from build123d import *

# Parameters (mm, degrees)
ESQUISSE1_R             = 24
BOSS_EXTRU_1_DEPTH      = 14
BOSS_EXTRU_2_DEPTH      = 8
ESQUISSE3_R             = 1.75
ENL_V_MAT_EXTRU_1_DEPTH = 8
BOSS_EXTRU_3_DEPTH      = 40
ESQUISSE5_R             = 17
BOSS_EXTRU_4_DEPTH      = 28
ESQUISSE6_R             = 13
ENL_V_MAT_EXTRU_2_DEPTH = 4
CHANFREIN1_SIZE         = 1


with BuildPart() as part:
    # Esquisse1 → Boss.-Extru.1 (new body)
    with BuildSketch(Plane(origin=(0, 0, 0), x_dir=(0, 0, -1), z_dir=(1, 0, 0))):
        Circle(ESQUISSE1_R)
    extrude(amount=BOSS_EXTRU_1_DEPTH)

    # Esquisse2 → Boss.-Extru.2 (add)
    with BuildSketch(Plane(origin=(14, 0, 0), x_dir=(0, 0, -1), z_dir=(1, 0, 0))):
        with BuildLine():
            Line((-32, -24), (32, -24))
            ThreePointArc((32, -24), (36.242640687, -22.242640687), (38, -18))
            Line((38, -18), (38, 18))
            ThreePointArc((38, 18), (36.242640687, 22.242640687), (32, 24))
            Line((32, 24), (-32, 24))
            ThreePointArc((-32, 24), (-36.242640687, 22.242640687), (-38, 18))
            Line((-38, 18), (-38, -18))
            ThreePointArc((-38, -18), (-36.242640687, -22.242640687), (-32, -24))
        make_face()
    extrude(amount=BOSS_EXTRU_2_DEPTH)

    # Esquisse3 → Enlèv. mat.-Extru.1 (cut)
    with BuildSketch(Plane(origin=(22, 0, 0), x_dir=(0, 0, -1), z_dir=(1, 0, 0))):
        with Locations((31, 17)):
            Circle(ESQUISSE3_R)
        with Locations((-31, 17)):
            Circle(ESQUISSE3_R)
        with Locations((-31, -17)):
            Circle(ESQUISSE3_R)
        with Locations((31, -17)):
            Circle(ESQUISSE3_R)
    extrude(amount=-ENL_V_MAT_EXTRU_1_DEPTH, mode=Mode.SUBTRACT)

    # Esquisse4 → Boss.-Extru.3 (add)
    with BuildSketch(Plane(origin=(22, 0, 0), x_dir=(0, 0, -1), z_dir=(1, 0, 0))):
        with BuildLine():
            Line((-22, -20), (22, -20))
            ThreePointArc((22, -20), (25.535533906, -18.535533906), (27, -15))
            Line((27, -15), (27, 15))
            ThreePointArc((27, 15), (25.535533906, 18.535533906), (22, 20))
            Line((22, 20), (-22, 20))
            ThreePointArc((-22, 20), (-25.535533906, 18.535533906), (-27, 15))
            Line((-27, 15), (-27, -15))
            ThreePointArc((-27, -15), (-25.535533906, -18.535533906), (-22, -20))
        make_face()
    extrude(amount=BOSS_EXTRU_3_DEPTH)

    # Esquisse5 → Boss.-Extru.4 (add)
    with BuildSketch(Plane(origin=(62, 0, 0), x_dir=(0, 0, -1), z_dir=(1, 0, 0))):
        Circle(ESQUISSE5_R)
    extrude(amount=BOSS_EXTRU_4_DEPTH)

    # Esquisse6 → Enlèv. mat.-Extru.2 (cut)
    with BuildSketch(Plane(origin=(90, 0, 0), x_dir=(0, 0, -1), z_dir=(1, 0, 0))):
        Circle(ESQUISSE6_R)
    extrude(amount=-ENL_V_MAT_EXTRU_2_DEPTH, mode=Mode.SUBTRACT)

    # Chanfrein1
    chanfrein1_edges = [part.edges().sort_by_distance(p)[0] for p in [
        (90, 0, 17),
    ]]
    chamfer(chanfrein1_edges, length=CHANFREIN1_SIZE)


solid = part.part
Could you check a few things on this model? Use its own coordinates, in mm. A direction names the side the tool comes from. Give positions to 0.01 mm unless a question says otherwise; leave off trailing zeros. Write each loop counter-clockwise with the first axis right and the second up, starting at its lowest first coordinate (ties: lowest second). Pieces come first, ordered by that corner, then holes. Notation, with made-up numbers: (-8, 77.25) - (19, 77.25) arc R19 cw to (19, 84.25) - close; hole circle Ø9 at (42, 89). An arc over 180 degrees is marked (long way). Use CSV: the item, a comma, the result in double quotes. Start each with the question number.
Item 1: For faces 1 (the face through (86, 0, 0)), 2 (the face through (42, 0, -27)), 3 (the face through (14, 0, 28)), which set-ups out of +Z, -Z, +X, -X, +Y, -Y let a thin tool reach every point of the face, with its end or its side?
Item 2: If I drill on line 1 along Y through (x, z) = (20.5, -31); line 2 along Y through (x, z) = (88, 0); line 3 along Y through (x, z) = (4, 0), over which ranges is the centre line in solid material (lowest first)?
Item 3: I'm going to push flat-ended pins straight in: pin 1 (12 mm diameter, centred on x = 50.5, z = 9, fed in from -Y); pin 2 (8 mm diameter, centred on x = 34.5, y = -18, fed in from +Z); pin 3 (10 mm diameter, centred on y = 16, z = 15.5, fed in from +X). Where does each tip first touch, or does it pass through?
Item 4: I want a section at A-A, the plane x = 43.5. Please give me the cut outline in (y, z), then the cut area to 3 significant figures.
Item 5: If we mould it in two halves opening along X, with no side actions, what happens to faces 4 (the face through (90, 13.1, 1.3)), 5 (the face through (0, 0, 0)), 6 (the face through (17.944, 22.196, -36.289))? For each: pulls with the +X half, pulls with the -X half, needs draft (parallel to the pull), parting line crosses it, or undercut.
Item 6: I want a section at B-B, the plane x = 72.5. Please give me the cut outline in (y, z).
Findings:
1,face 1,"+X"
1,face 2,"-Z, +X, +Y, -Y"
1,face 3,"+Z, -X"
2,line 1,"y = -24 to -18.75, -15.25 to 15.25, 18.75 to 24"
2,line 2,"y = -17 to -13, 13 to 17"
2,line 3,"y = -24 to 24"
3,pin 1,"stops at y = -20"
3,pin 2,"stops at z = 27"
3,pin 3,"stops at x = 62"
4,outline,"(-20, -22) arc R5 ccw to (-15, -27) - (15, -27) arc R5 ccw to (20, -22) - (20, 22) arc R5 ccw to (15, 27) - (-15, 27) arc R5 ccw to (-20, 22) - close"
4,area,"2,140 mm2"
5,face 4,"pulls with the +X half"
5,face 5,"pulls with the -X half"
5,face 6,"needs draft"
6,outline,"circle Ø34 at (0, 0)"
